Autodesk Inventor part; units mm, degrees
ref_plane "MSC_PF1" through (0, 0, 0) normal (1, 0, 0) x (0, 1, 0)
ref_plane "MSC_PT1" through (0, 0, 0) normal (0, 0, -1) x (-1, 0, 0)
ref_plane "YZ Plane" through (0, 0, 0) normal (1, 0, 0) x (0, 1, 0)
sketch "Skizze1" plane through (0, 0, 0) normal (0, 1, 0) x (-1, 0, 0)
  point P0 (0, 0)
sketch "Skizze2" plane through (0, 0, 0) normal (0, 0, 1) x (1, 0, 0)
  point P0 (0, 0)
sketch "Skizze3" plane through (0, 0, 0) normal (0, 0, 1) x (1, 0, 0)
  point P0 (0, 0)
sketch "Skizze4" plane through (0, 0, 0) normal (0, 1, 0) x (-1, 0, 0)
  line L0 (-1.9, 0) -> (0, 0)
  line L1 (-1.9, -0.3) -> (-1.9, 0)
  line L2 (-1, -1.2) -> (-1.9, -0.3)
  line L3 (-1, -1.6) -> (-1, -1.2)
  line L4 (-0.8, -1.8) -> (-1, -1.6)
  line L5 (-1, -2.2) -> (-0.8, -1.8)
  line L6 (-1, -6) -> (-1, -2.2)
  line L7 (0, 0) -> (0, -6)
  line L8 (0, 3.3392) -> (0, -10.7) construction
  line L9 (0, 3.3392) -> (0, -10.7)
  line L10 (0, -13.5078) -> (0, 6.1471)
  line L11 (-1, -6) -> (0, -6)
  line L12 (0.38, 0) -> (-2.28, 0)
  dimension "d3" = 1.9
  dimension "d5" = 0.4
  dimension "d7" = 0.2
  dimension "d9" = 0.4
  dimension "d11" = 1.2
  dimension "d13" = 135
  dimension "d17" = 0.8
  dimension "d19" = 0
  dimension "d51" = 1
  dimension "d52" = 6
revolve "Drehung1" add sketch "Skizze4" angle 360 about axis through (0, 0, 3.3392) along (0, 0, -1)
sketch "Skizze5" plane through (0, 0, 0) normal (0, 1, 0) x (-1, 0, 0)
  line L0 (-0.95, 0) -> (0, 0)
  line L1 (-0.1583, -1.0909) -> (-0.95, 0)
  line L2 (0, -1.0909) -> (-0.1583, -1.0909)
  line L3 (0, 0) -> (0, -1.0909)
  line L4 (-1, -1.2) -> (1, -1.2) construction
  line L5 (-1.9, 0) -> (1.9, 0)
  line L6 (0, -1.44) -> (0, 0.24)
  dimension "d22" = 0.95
  dimension "d24" = 0.1583
  dimension "d26" = 1.0909
extrude "Extrusion1" cut sketch "Skizze5" along normal mid plane 0.3167
pattern_circular "Polare Anordnung1" count 4 over 360 about axis through (0, 0, 0) along (0, 0, 1) of "Extrusion1"
sketch "Skizze7" plane through (0, 0, 0) normal (0, 1, 0) x (-1, 0, 0)
  line L0 (0, -0.6) -> (-1.1875, 0)
  line L1 (0, 0) -> (0, -0.6)
  line L2 (-1.1875, 0) -> (0, 0)
  line L3 (-1, -1.2) -> (1, -1.2) construction
  line L4 (0, -1.44) -> (0, 0.24)
  line L5 (-1.9, 0) -> (1.9, 0)
  dimension "d33" = 1.1875
  dimension "d35" = 0.6
extrude "Extrusion2" cut sketch "Skizze7" along normal mid plane 0.3167
pattern_circular "Polare Anordnung2" count 4 over 360 about axis through (0, 0, 0) along (0, 0, 1) of "Extrusion2"
fillet "Rundung1" radius 0.8 1 edges at (-1, 0, -1.2)
thread "Gewinde1"
ref_plane "MSC_PF1" through (0, 0, 0) normal (1, 0, 0) x (0, 1, 0)
ref_plane "MSC_PT1" through (0, 0, 0) normal (0, 0, -1) x (-1, 0, 0)
equation "\"d3\" = 0.5 * Dh"
equation "\"d5\" = msp_x"
equation "\"d7\" = ParA"
equation "\"d9\" = msp_x"
equation "\"d11\" = ParK"
equation "\"d17\" = 0.5 * msp_mdtds"
equation "\"d51\" = 0.5 * NND"
equation "\"d52\" = NLG"
equation "\"d22\" = 0.5 * M"
equation "\"d24\" = 0.0833333 * M"
equation "\"d26\" = 0.909091 * ParK"
equation "\"d27\" = 0.166667 * M"
equation "\"d33\" = 0.625 * M"
equation "\"d35\" = 0.5 * ParK"
equation "\"d36\" = 0.166667 * M"
equation "\"d41\" = 2 * msp_x"
equation "\"PTC\" = 0.4"
equation "\"NLG\" = 6"
equation "\"ParK\" = 1.2"
equation "\"NND\" = 2"
equation "\"M\" = 1.9"
equation "\"msp_mdtds\" = NND - PTC"
equation "\"Dh\" = 3.8"
equation "\"msp_x\" = PTC"
equation "\"ParA\" = 0.5 * PTC"
equation "\"r\" = 0.5"
equation "\"THREADDIA\" = NND"
equation "\"TEMPLATE\" = 1.2345"
properties part number "DIN EN ISO 7046-2 H - M2x6 - 8.8 - H1" material "Stahl"
Geometry: final body of the model. Coordinates: model frame, mm. A direction names the side the tool comes from. Give positions to 0.01 mm unless a question says otherwise; leave off trailing zeros. Loops run counter-clockwise (first coordinate to the right, second up) from the corner with the lowest first, then second, coordinate; pieces in that order, holes last. Notation, with made-up numbers: M 61,57.25 L 88,57.25 A27 ccw 88,81.25 Z; hole C -32,7 d3. An arc over 180 degrees is marked long. Put each result on its own line as item: value. Start each with the question number.
1) Ray query, line 1 along Z through (x, y) = (0.7, -1.2); line 2 along Z through (x, y) = (-0.9, 0.1); line 3 along Z through (x, y) = (1.2, 0.1). Return the intervals inside material, ascending.
2) Access query for faces 1 (the flat face through (0, 0, -6)), 2 (the cylindrical face through (0, -1, -4)), 3 (the flat face through (0.5, -0.158, -0.3)). Directions: +Z, -Z, +X, -X, +Y, -Y. A direction counts if a zero-diameter tool reaches every point of the face in a straight line with its end or side. Return the directions, or none.
3) Contact query for flat-ended pins moving along their axis: pin 1 (1 mm diameter, centred on x = 1, y = -1, fed in from +Z); pin 2 (0.8 mm diameter, centred on x = 0.5, z = -0.5, fed in from +Y); pin 3 (1.1 mm diameter, centred on x = -1, z = -0.5, fed in from -Y); pin 4 (1.1 mm diameter, centred on x = -1, z = -0.5, fed in from +Y). Output: stop coordinate, or through.
4) Cut plane B-B (z = -2). Output: boundary loops of the cut face in (x, y).
5) Cut plane A-A (z = -0.65). Output: boundary loops of the cut face in (x, y), then the cut area to 3 significant figures.
6) Cut plane C-C (z = -5.05). Output: boundary loops of the cut face in (x, y).
Verdict:
1. line 1: -0.81 to 0
1. line 2: -6 to -2.01, -1.69 to -0.15
1. line 3: -1 to 0
2. face 1: -Z, +X, -X, +Y, -Y
2. face 2: -Z
2. face 3: +Z
3. pin 1: z = 0
3. pin 2: y = 1.89
3. pin 3: y = -1.84
3. pin 4: y = 1.84
4. outline: C 0,0 d1.8
5. outline: C 0,0 d3.1; hole M -0.48,-0.16 L -0.16,-0.16 L -0.16,-0.48 L 0.16,-0.48 L 0.16,-0.16 L 0.48,-0.16 L 0.48,0.16 L 0.16,0.16 L 0.16,0.48 L -0.16,0.48 L -0.16,0.16 L -0.48,0.16 Z
5. area: 7.04 mm2
6. outline: C 0,0 d2
